Check sheet for the modelled part. Datum: model origin and axes. Units: mm. Give positions to 0.01 mm unless a question says otherwise; leave off trailing zeros. Order: outer loops, then holes, each group sorted by start corner. A loop starts at its lowest first (then second) coordinate and runs counter-clockwise, first axis right, second up. Notation, with made-up numbers: (1.25, 32) -> (18.25, 32) arc R23 ccw to (18.25, 47) -> close; hole circle Ø8 at (2.5, 25). An arc over 180 degrees is marked (long way). Write each question's results on one line, items separated by ' | '.
from build123d import *

# Parameters (mm, degrees)
SKETCH1_R           = 5.715
BOSS_EXTRUDE1_DEPTH = 4.445
FILLET2_R           = 0.254
SKETCH2_W           = 2.54
SKETCH2_H           = 5.715
CUT_EXTRUDE1_DEPTH  = 10.223907794
BOSS_EXTRUDE2_DEPTH = 4.572


with BuildPart() as part:
    # Sketch1 → Boss-Extrude1 (new body)
    with BuildSketch(Plane(origin=(0, 0, 0), x_dir=(1, 0, 0), z_dir=(0, 1, 0))):
        with Locations(Location((0, 0, 0), (0, 0, 270))):
            Circle(SKETCH1_R)
    extrude(amount=BOSS_EXTRUDE1_DEPTH)

    # Fillet2
    fillet2_edges = [part.edges().sort_by_distance(p)[0] for p in [
        (0, 4.445, -5.715),
    ]]
    fillet(fillet2_edges, radius=FILLET2_R)

    # Sketch2 → Cut-Extrude1 (cut, through all)
    with BuildSketch(Plane.XZ):
        with Locations((0, 2.8575)):
            Rectangle(SKETCH2_W, SKETCH2_H)
    extrude(amount=-CUT_EXTRUDE1_DEPTH, mode=Mode.SUBTRACT)

    # Sketch3 → Boss-Extrude2 (add)
    with BuildSketch(Plane.XZ):
        with BuildLine():
            Line((-1.27, 0), (-1.27, 5.572102386))
            ThreePointArc((-1.27, 5.572102386), (0, 5.715), (1.27, 5.572102386))
            Line((1.27, 5.572102386), (1.27, 0))
            Line((1.27, 0), (-1.27, 0))
        make_face()
    extrude(amount=-BOSS_EXTRUDE2_DEPTH)


solid = part.part
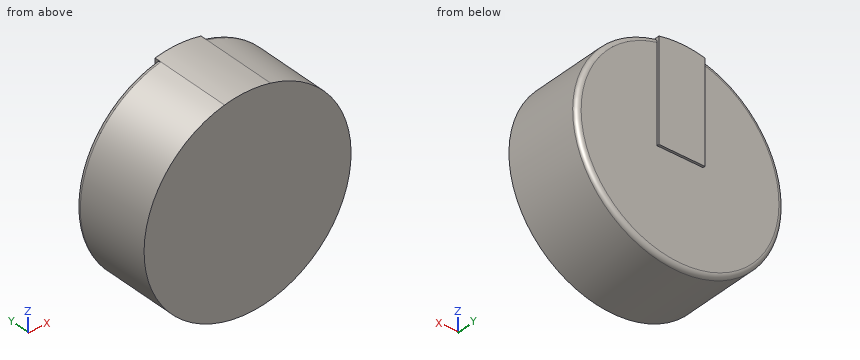
1. Gauge pin test, flat ends, axial feed: pin 1 Ø1 at (y, z) = (3, -3.5) entering from -X; pin 2 Ø1 at (x, y) = (-1, 2) entering from +Z. Record the tip position at first contact, or that the pin passes through.
Verdict:
pin 1: stops at x = -4.86 | pin 2: stops at z = 5.69
2. Material ranges on probe 1 along Y at (x, z) = (1.5, -3.75) (3 decimals); probe 2 along Z at (x, y) = (-1.5, 4.1); probe 3 along Z at (x, y) = (3, 0.55), recorded low to high. Write a range as from..to.
Verdict:
probe 1: y = 0..4.445 | probe 2: z = -5.51..5.51 | probe 3: z = -4.86..4.86
3. Section check A-A on y = 3.9. Record the cut outline in (x, z) (3 decimals).
Verdict:
outline: circle Ø11.43 at (0, 0)
